from build123d import *

# Parameters (mm, degrees)
SKETCH_1_W           = 89
SKETCH_1_H           = 37.5
EXTRUDE_1_DEPTH      = 8
SKETCH_2_W           = 85
SKETCH_2_H           = 33.5
CUT_EXTRUDE_1_DEPTH  = 6.5
FILLET_2_R           = 2
FILLET_3_R           = 2
FILLET_4_R           = 2
FILLET_5_R           = 2
FILLET_6_R           = 2
FILLET_7_R           = 2
SKETCH_3_R           = 2.5
SKETCH_3_W           = 10
SKETCH_3_H           = 2
SKETCH_3_W_2         = 3
SKETCH_3_H_2         = 17.5
EXTRUDE_2_DEPTH      = 5.5
SKETCH_4_R           = 0.8
CUT_EXTRUDE_2_DEPTH  = 97.831038412
SKETCH_5_R           = 0.8
CUT_EXTRUDE_3_DEPTH  = 97.831038412
SKETCH_6_R           = 0.8
CUT_EXTRUDE_4_DEPTH  = 97.831038412
SKETCH_8_R           = 0.8
CUT_EXTRUDE_5_DEPTH  = 97.831038412
SKETCH_9_R           = 2
CUT_EXTRUDE_6_DEPTH  = 1
CUT_EXTRUDE_7_DEPTH  = 2
SKETCH_11_W          = 8.8
SKETCH_11_H          = 4
CUT_EXTRUDE_8_DEPTH  = 2
SKETCH_12_W          = 11.8
SKETCH_12_H          = 4
CUT_EXTRUDE_9_DEPTH  = 1
CUT_EXTRUDE_10_DEPTH = 6.5
EXTRUDE_3_DEPTH      = 3.5
CUT_EXTRUDE_START    = -1.5
CUT_EXTRUDE_12_DEPTH = 1.5
SKETCH_18_W          = 10
SKETCH_18_H          = 3.5
CUT_EXTRUDE_15_DEPTH = 1


with BuildPart() as part:
    # 草图1 → 凸台-拉伸1 (new body)
    with BuildSketch(Plane.XY):
        with Locations((44.5, -18.75)):
            Rectangle(SKETCH_1_W, SKETCH_1_H)
    extrude(amount=EXTRUDE_1_DEPTH)

    # 草图2 → 切除-拉伸1 (cut)
    with BuildSketch(Plane.XY.offset(8)):
        with Locations((44.5, -18.75)):
            Rectangle(SKETCH_2_W, SKETCH_2_H)
    extrude(amount=-CUT_EXTRUDE_1_DEPTH, mode=Mode.SUBTRACT)

    # 圆角2
    fillet_2_edges = [part.edges().sort_by_distance(p)[0] for p in [
        (44.5, 0, 0),
        (89, -18.75, 0),
        (44.5, -37.5, 0),
        (0, -18.75, 0),
    ]]
    fillet(fillet_2_edges, radius=FILLET_2_R)

    # 圆角3
    fillet_3_edges = [part.edges().sort_by_distance(p)[0] for p in [
        (87, -35.5, 4.75),
    ]]
    fillet(fillet_3_edges, radius=FILLET_3_R)

    # 圆角4
    fillet_4_edges = [part.edges().sort_by_distance(p)[0] for p in [
        (87, -2, 4.75),
    ]]
    fillet(fillet_4_edges, radius=FILLET_4_R)

    # 圆角5
    fillet_5_edges = [part.edges().sort_by_distance(p)[0] for p in [
        (2, -35.5, 4.75),
    ]]
    fillet(fillet_5_edges, radius=FILLET_5_R)

    # 圆角6
    fillet_6_edges = [part.edges().sort_by_distance(p)[0] for p in [
        (2, -2, 4.75),
    ]]
    fillet(fillet_6_edges, radius=FILLET_6_R)

    # 圆角7
    # the kernel refuses this fillet: 2 mm, written as the material it takes off along each edge
    with BuildSketch(Plane(origin=(2, -2, 2), x_dir=(-1, 0, 0), z_dir=(0, 1, 0))) as fillet_7_piece_1_section:
        Polygon((0, 0), (FILLET_7_R, 0), (FILLET_7_R, -FILLET_7_R), (0, -FILLET_7_R), align=None)
    fillet_7_piece_1 = extrude(amount=FILLET_7_R, mode=Mode.PRIVATE)
    fillet_7_piece_1 = fillet_7_piece_1 - Plane(origin=(2, -2, 2), x_dir=(0.7071067811865475, 0, 0.7071067811865475), z_dir=(0, 1, 0)) * Sphere(FILLET_7_R, mode=Mode.PRIVATE)
    add(fillet_7_piece_1, mode=Mode.SUBTRACT)
    with BuildSketch(Plane(origin=(87, -2, 2), x_dir=(1, 0, 0), z_dir=(0, 1, 0))) as fillet_7_piece_2_section:
        Polygon((0, 0), (FILLET_7_R, 0), (FILLET_7_R, FILLET_7_R), (0, FILLET_7_R), align=None)
    fillet_7_piece_2 = extrude(amount=FILLET_7_R, mode=Mode.PRIVATE)
    fillet_7_piece_2 = fillet_7_piece_2 - Plane(origin=(87, -2, 2), x_dir=(-0.7071067811865475, 0, 0.7071067811865475), z_dir=(0, 1, 0)) * Sphere(FILLET_7_R, mode=Mode.PRIVATE)
    add(fillet_7_piece_2, mode=Mode.SUBTRACT)
    with BuildSketch(Plane(origin=(2, -35.5, 2), x_dir=(0, -1, 0), z_dir=(-1, 0, 0))) as fillet_7_piece_3_section:
        Polygon((0, 0), (FILLET_7_R, 0), (FILLET_7_R, -FILLET_7_R), (0, -FILLET_7_R), align=None)
    fillet_7_piece_3 = extrude(amount=FILLET_7_R, mode=Mode.PRIVATE)
    fillet_7_piece_3 = fillet_7_piece_3 - Plane(origin=(2, -35.5, 2), x_dir=(0, 0.7071067811865475, 0.7071067811865475), z_dir=(-1, 0, 0)) * Sphere(FILLET_7_R, mode=Mode.PRIVATE)
    add(fillet_7_piece_3, mode=Mode.SUBTRACT)
    with BuildSketch(Plane(origin=(87, -35.5, 2), x_dir=(0, -1, 0), z_dir=(1, 0, 0))) as fillet_7_piece_4_section:
        Polygon((0, 0), (FILLET_7_R, 0), (FILLET_7_R, FILLET_7_R), (0, FILLET_7_R), align=None)
    fillet_7_piece_4 = extrude(amount=FILLET_7_R, mode=Mode.PRIVATE)
    fillet_7_piece_4 = fillet_7_piece_4 - Plane(origin=(87, -35.5, 2), x_dir=(0, 0.7071067811865475, 0.7071067811865475), z_dir=(1, 0, 0)) * Sphere(FILLET_7_R, mode=Mode.PRIVATE)
    add(fillet_7_piece_4, mode=Mode.SUBTRACT)
    with BuildSketch(Plane(origin=(0, 0, 2), x_dir=(1, 0, 0), z_dir=(0, 0, 1)), Plane(origin=(0, -37.5, 2), x_dir=(0, 1, 0), z_dir=(0, 0, 1))) as fillet_7_piece_5:
        with BuildLine():
            CenterArc((FILLET_7_R, -FILLET_7_R), FILLET_7_R, 90, 90)
            Line((0, -FILLET_7_R), (0, 0))
            Line((0, 0), (FILLET_7_R, 0))
        make_face()
    extrude(amount=11, mode=Mode.SUBTRACT)
    with BuildSketch(Plane(origin=(89, 0, 2), x_dir=(-1, 0, 0), z_dir=(0, 0, 1)), Plane(origin=(89, -37.5, 2), x_dir=(0, 1, 0), z_dir=(0, 0, 1))) as fillet_7_piece_6:
        with BuildLine():
            CenterArc((FILLET_7_R, FILLET_7_R), FILLET_7_R, 180, 90)
            Line((0, FILLET_7_R), (0, 0))
            Line((0, 0), (FILLET_7_R, 0))
        make_face()
    extrude(amount=11, mode=Mode.SUBTRACT)

    # 草图3 → 凸台-拉伸2 (add)
    with BuildSketch(Plane.XY.offset(1.5)):
        with Locations((83.8, -5.4)):
            Circle(SKETCH_3_R)
        with Locations((83.8, -32.1)):
            Circle(SKETCH_3_R)
        with Locations((10, -5.4)):
            Circle(SKETCH_3_R)
        with Locations((10, -32.053618844)):
            Circle(SKETCH_3_R)
        with Locations((62, -3)):
            Rectangle(SKETCH_3_W, SKETCH_3_H)
        with Locations((27, -34.5)):
            Rectangle(SKETCH_3_W, SKETCH_3_H)
        with Locations((80.5, -18.75)):
            Rectangle(SKETCH_3_W_2, SKETCH_3_H_2)
        with Locations((33.5, -18.75)):
            Rectangle(SKETCH_3_W_2, SKETCH_3_H_2)
    extrude(amount=EXTRUDE_2_DEPTH)

    # 草图4 → 切除-拉伸2 (cut, through all)
    with BuildSketch(Plane.XY.offset(7)):
        with Locations((10, -5.4)):
            Circle(SKETCH_4_R)
    extrude(amount=-CUT_EXTRUDE_2_DEPTH, mode=Mode.SUBTRACT)

    # 草图5 → 切除-拉伸3 (cut, through all)
    with BuildSketch(Plane.XY.offset(7)):
        with Locations((83.8, -5.4)):
            Circle(SKETCH_5_R)
    extrude(amount=-CUT_EXTRUDE_3_DEPTH, mode=Mode.SUBTRACT)

    # 草图6 → 切除-拉伸4 (cut, through all)
    with BuildSketch(Plane.XY.offset(7)):
        with Locations((10, -32.053618844)):
            Circle(SKETCH_6_R)
    extrude(amount=-CUT_EXTRUDE_4_DEPTH, mode=Mode.SUBTRACT)

    # 草图8 → 切除-拉伸5 (cut, through all)
    with BuildSketch(Plane.XY.offset(7)):
        with Locations((83.8, -32.1)):
            Circle(SKETCH_8_R)
    extrude(amount=-CUT_EXTRUDE_5_DEPTH, mode=Mode.SUBTRACT)

    # 草图9 → 切除-拉伸6 (cut)
    with BuildSketch(Plane(origin=(0, 0, 0), x_dir=(-1, 0, 0), z_dir=(0, 0, -1))):
        with Locations((-83.8, -5.4)):
            Circle(SKETCH_9_R)
        with Locations((-10, -5.4)):
            Circle(SKETCH_9_R)
        with Locations((-10, -32.053618844)):
            Circle(SKETCH_9_R)
        with Locations((-83.8, -32.1)):
            Circle(SKETCH_9_R)
    extrude(amount=-CUT_EXTRUDE_6_DEPTH, mode=Mode.SUBTRACT)

    # 草图10 → 切除-拉伸7 (cut)
    with BuildSketch(Plane.ZY):
        with BuildLine():
            Line((8, -17.15), (8, -20.35))
            ThreePointArc((8, -20.35), (6.4, -18.75), (8, -17.15))
        make_face()
    extrude(amount=-CUT_EXTRUDE_7_DEPTH, mode=Mode.SUBTRACT)

    # 草图11 → 切除-拉伸8 (cut)
    with BuildSketch(Plane.XZ.offset(37.5)):
        with Locations((72.8, 4)):
            Rectangle(SKETCH_11_W, SKETCH_11_H)
        with Locations((47.5, 4)):
            Rectangle(SKETCH_11_W, SKETCH_11_H)
    extrude(amount=-CUT_EXTRUDE_8_DEPTH, mode=Mode.SUBTRACT)

    # 草图12 → 切除-拉伸9 (cut)
    with BuildSketch(Plane(origin=(0, -35.5, 0), x_dir=(1, 0, 0), z_dir=(0, 1, 0))):
        with Locations((72.8, -4)):
            Rectangle(SKETCH_12_W, SKETCH_12_H)
        with Locations((47.5, -4)):
            Rectangle(SKETCH_12_W, SKETCH_12_H)
    extrude(amount=-CUT_EXTRUDE_9_DEPTH, mode=Mode.SUBTRACT)

    # 草图13 → 切除-拉伸10 (cut)
    with BuildSketch(Plane.XY.offset(8)):
        Polygon((29.8, 0), (30.8, -2), (15.8, -2), (16.8, 0), align=None)
    extrude(amount=-CUT_EXTRUDE_10_DEPTH, mode=Mode.SUBTRACT)

    # 草图14 → 凸台-拉伸3 (add)
    with BuildSketch(Plane.XY.offset(8)):
        Polygon((15.8, -2), (16.8, 0), (29.8, 0), (30.8, -2), align=None)
    extrude(amount=-EXTRUDE_3_DEPTH)

    # 草图15 → 切除-拉伸12 (cut)
    with BuildSketch(Plane.XY.offset(8).offset(CUT_EXTRUDE_START)):
        with BuildLine():
            Line((2, 0), (87, 0))
            ThreePointArc((87, 0), (88.414213562, -0.585786438), (89, -2))
            Line((89, -2), (89, -35.5))
            ThreePointArc((89, -35.5), (88.414213562, -36.914213562), (87, -37.5))
            Line((87, -37.5), (2, -37.5))
            ThreePointArc((2, -37.5), (0.585786438, -36.914213562), (0, -35.5))
            Line((0, -35.5), (0, -20.35))
            Line((0, -20.35), (1, -20.35))
            Line((1, -20.35), (1, -34.5))
            ThreePointArc((1, -34.5), (1.585786438, -35.914213562), (3, -36.5))
            Line((3, -36.5), (86, -36.5))
            ThreePointArc((86, -36.5), (87.414213562, -35.914213562), (88, -34.5))
            Line((88, -34.5), (88, -3))
            ThreePointArc((88, -3), (87.414213562, -1.585786438), (86, -1))
            Line((86, -1), (3, -1))
            ThreePointArc((3, -1), (1.585786438, -1.585786438), (1, -3))
            Line((1, -3), (1, -17.15))
            Line((1, -17.15), (0, -17.15))
            Line((0, -17.15), (0, -2))
            ThreePointArc((0, -2), (0.585786438, -0.585786438), (2, 0))
        make_face()
    extrude(amount=CUT_EXTRUDE_12_DEPTH, mode=Mode.SUBTRACT)

    # 草图18 → 切除-拉伸15 (cut)
    with BuildSketch(Plane(origin=(0, -2, 0), x_dir=(-1, 0, 0), z_dir=(0, -1, 0))):
        with Locations((-23.3, -6.25)):
            Rectangle(SKETCH_18_W, SKETCH_18_H)
    extrude(amount=-CUT_EXTRUDE_15_DEPTH, mode=Mode.SUBTRACT)


solid = part.part
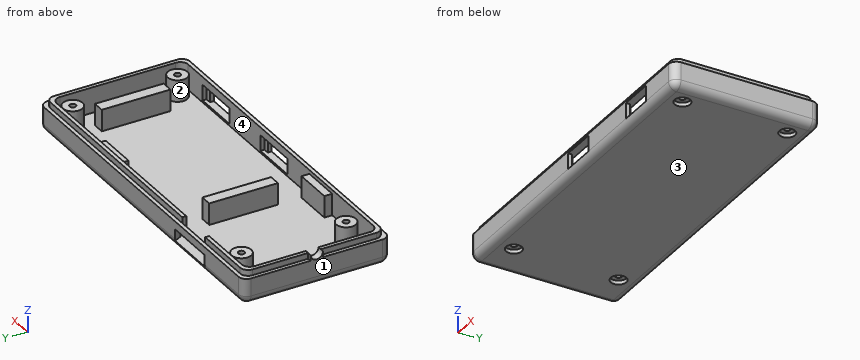
Verification items for the finished model (mm, model axes). Face numbers are marked on the shaded views. A direction names the side the tool comes from. Give positions to 0.01 mm unless a question says otherwise; leave off trailing zeros. Order: outer loops, then holes, each group sorted by start corner. A loop starts at its lowest first (then second) coordinate and runs counter-clockwise, first axis right, second up. Notation, with made-up numbers: M 37,87 L 78,87 A15 ccw 78,103 Z; hole C 65.5,15 d5. An arc over 180 degrees is marked long. Answer as a JSON object with one key per item and string values. Group by question number.
1) Cross-section at B-B (x = 6.5). Enter the section's corners in (y, z).
2) Mould release check, pull along Y, two halves, no side actions. Record for the marked faces 3 and 4: released by +Y, released by -Y, zero draft, split by the parting line, or undercut.
3) Depth check by flat-ended pin: pin 1 Ø3 at (x, y) = (83.8, -32.1) entering from -Z; pin 2 Ø0.6 at (x, y) = (24, -0.5) entering from -Z; pin 3 Ø3.5 at (x, y) = (83.8, -5.4) entering from +Z. Enter the tip coordinate at first touch or a pass-through.
4) Cross-section at C-C (x = 83.8). Give the number of separate pieces and of enclosed holes in the cut face, then the cut area to 3 significant figures.
5) Cross-section at A-A (y = -26.5). Enter the section's corners in (x, z), then the cut area to 3 significant figures.
6) Access from +Z, -Z, +X, -X, +Y, -Y to the whole of each face (thin tool, end or side, straight path). Record for the marked faces 1 and 2.
7) Scan lines: line 1 along X through (y, z) = (-27, 4); line 2 along Y through (x, z) = (83.8, 4.15); line 3 along Y through (x, z) = (6.5, 3.5). Record each from-to range of solid material in increasing order. Write a range as [from, to].
Result sheet:
{
 "1": {"outline": "M -37.5,2 A2 ccw -35.5,0 L -2,0 A2 ccw 0,2 L 0,6.5 L -1,6.5 L -1,8 L -2,8 L -2,1.5 L -35.5,1.5 L -35.5,8 L -36.5,8 L -36.5,6.5 L -37.5,6.5 Z"},
 "2": {"face 3": "zero draft", "face 4": "undercut"},
 "3": {"pin 1": "stops at z = 1", "pin 2": "stops at z = 0.4", "pin 3": "stops at z = 7"},
 "4": {"separate pieces": "3", "enclosed holes": "0", "area": "105 mm2"},
 "5": {"outline": "M 0,2 A2 ccw 2,0 L 87,0 A2 ccw 89,2 L 89,6.5 L 88,6.5 L 88,8 L 87,8 L 87,1.5 L 82,1.5 L 82,7 L 79,7 L 79,1.5 L 35,1.5 L 35,7 L 32,7 L 32,1.5 L 2,1.5 L 2,8 L 1,8 L 1,6.5 L 0,6.5 Z", "area": "188 mm2"},
 "6": {"face 1": "+Z, -Z, -X, +Y, -Y", "face 2": "+Z"},
 "7": {"line 1": "x = [0, 2], [32, 35], [79, 82], [87, 89]", "line 2": "y = [-37.5, -35.5], [-34.6, -32.9], [-31.3, -29.6], [-7.9, -6.2], [-4.6, -2.9], [-2, 0]", "line 3": "y = [-37.5, -35.5], [-2, 0]"}
}
